Input: dimensioned drawing with shaded views. Units: mm. Origin: part minimum x, y, z. A direction names the side the tool comes from. Round coordinates to 2 decimals unless told otherwise and drop trailing zeros. Write each loop counter-clockwise with the first axis right and the second up, starting at its lowest first coordinate (ties: lowest second). Pieces come first, ordered by that corner, then holes. Notation, with made-up numbers: (64, 71) - (73, 71) arc R28 ccw to (73, 89) - close; hole circle Ø2 at (47.5, -32.5). An arc over 180 degrees is marked (long way). Use one line per item in the form item = value.
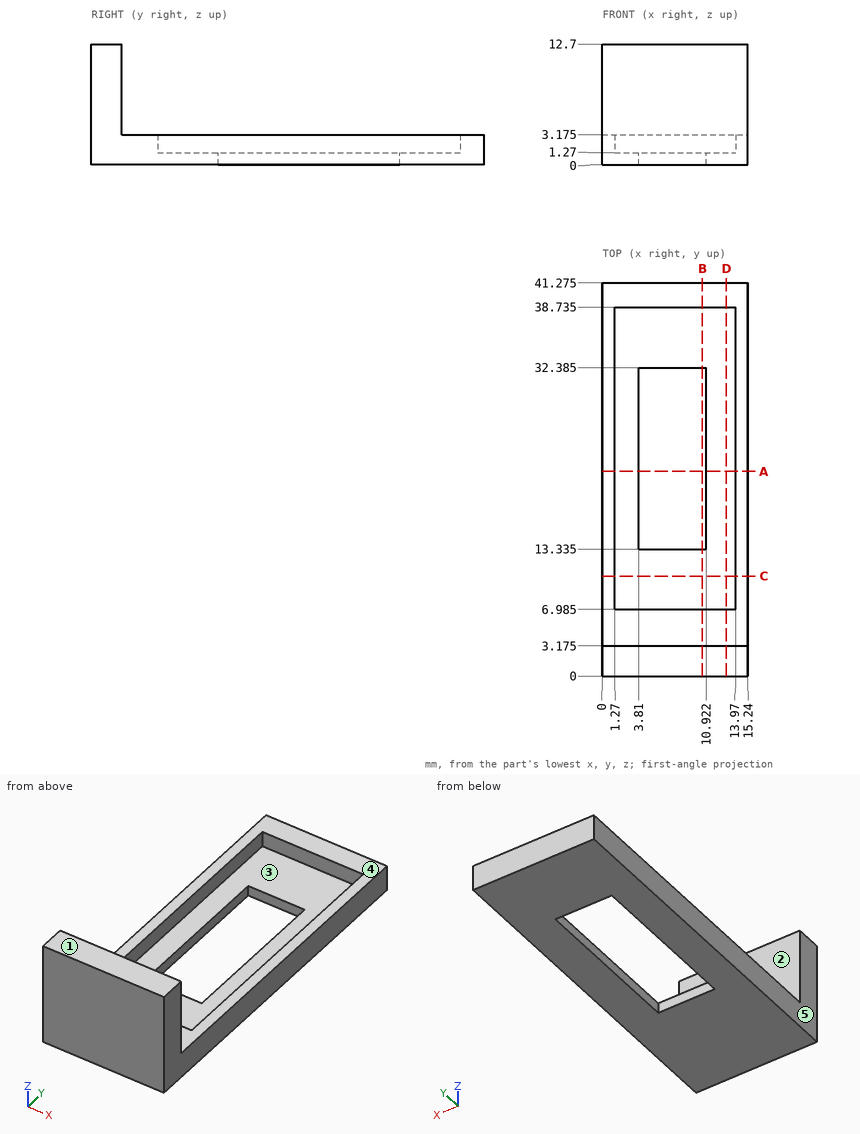
(1) Material intervals for L1, parallel to Y at x = 8, z = 1 (3 decimals); L2, parallel to Y at x = 7.75, z = 2.75 (3 decimals); L3, parallel to Z at x = 2.5, y = 29, sorted ascending.
Derived:
L1 = 0 to 13.335, 32.385 to 41.275
L2 = 0 to 6.985, 38.735 to 41.275
L3 = 0 to 1.27
(2) Draft query along X for the marked faces 3, 4 and 5. Return one class per face: released by +X, released by -X, zero draft, split by the parting line, or undercut.
Derived:
face_3 = undercut
face_4 = zero draft
face_5 = released by -X
(3) Cut plane A-A on y = 21.5. Output: boundary loops of the cut face in (x, z) (3 decimals), then the cut area to 3 significant figures.
Derived:
outline = (0, 0) - (3.81, 0) - (3.81, 1.27) - (1.27, 1.27) - (1.27, 3.175) - (0, 3.175) - close; (10.922, 0) - (15.24, 0) - (15.24, 3.175) - (13.97, 3.175) - (13.97, 1.27) - (10.922, 1.27) - close
area = 15.2 mm^2
(4) Cut plane C-C on y = 10.5. Output: boundary loops of the cut face in (x, z) (3 decimals), then the cut area to 3 significant figures.
Derived:
outline = (0, 0) - (15.24, 0) - (15.24, 3.175) - (13.97, 3.175) - (13.97, 1.27) - (1.27, 1.27) - (1.27, 3.175) - (0, 3.175) - close
area = 24.2 mm^2
(5) Cut plane B-B on x = 10.5. Output: boundary loops of the cut face in (y, z) (3 decimals).
Derived:
outline = (0, 0) - (13.335, 0) - (13.335, 1.27) - (6.985, 1.27) - (6.985, 3.175) - (3.175, 3.175) - (3.175, 12.7) - (0, 12.7) - close; (32.385, 0) - (41.275, 0) - (41.275, 3.175) - (38.735, 3.175) - (38.735, 1.27) - (32.385, 1.27) - close
(6) Cut plane D-D on x = 13. Output: boundary loops of the cut face in (y, z) (3 decimals), then the cut area to 3 significant figures.
Derived:
outline = (0, 0) - (41.275, 0) - (41.275, 3.175) - (38.735, 3.175) - (38.735, 1.27) - (6.985, 1.27) - (6.985, 3.175) - (3.175, 3.175) - (3.175, 12.7) - (0, 12.7) - close
area = 101 mm^2
(7) Access query for the marked faces 1 and 2. Directions: +Z, -Z, +X, -X, +Y, -Y. A direction counts if a zero-diameter tool reaches every point of the face in a straight line with its end or side. Return the directions, or none.
Derived:
face_1 = +Z, +X, -X, +Y, -Y
face_2 = +Z, +X, -X, +Y
(8) First-contact query: pin 1 Ø5 at (x, y) = (8, 13.5) entering from +Z; pin 2 Ø2 at (x, z) = (12, 11) entering from +Y (3 decimals). Flat tips, straight axial feed; report the tip coordinate or a pass-through.
Derived:
pin_1 = 1.27
pin_2 = 3.175
